```python
from build123d import *

# Parameters (mm, degrees)
CUT_SWEEP1_PITCH   = 0.793751588
CUT_EXTRUDE1_DEPTH = 1.955803912
FILLET1_R          = 0.30480061
FILLET2_R          = 0.396875794
CHAMFER3_SIZE      = 0.127


with BuildPart() as part:
    # Sketch1 → Revolve1 (revolve)
    with BuildSketch(Plane.XY, mode=Mode.PRIVATE) as revolve1_sk:
        Polygon((0, 0), (0, 29.565608331), (2.082804166, 29.565608331), (2.082804166, 4.165608331), (3.429006858, 4.165608331), (3.429006858, 0), align=None)
    revolve(revolve1_sk.sketch.rotate(Axis((0, 0, 0), (0, 1, 0)), 90), axis=Axis((0, 0, 0), (0, 1, 0)))

    # Cut-Sweep1: arcs per turn and ends read off the stored shape
    # Cut-Sweep1: the profile of Sketch3 profile screwed along a right-hand helix through 4.999992 turns, 8 arcs to a turn; built about Z, then put on its axis
    cut_sweep1_z = Axis((0, 0, 0), (0, 0, 1))
    cut_sweep1_corners = [(2.083104166, 0, -0.595163691), (2.083104166, 0, -0.992339484), (1.685928372, 0, -0.793751588)]
    with BuildLine(mode=Mode.PRIVATE) as cut_sweep1_profile:
        Line(cut_sweep1_corners[0], cut_sweep1_corners[1])
        Line(cut_sweep1_corners[1], cut_sweep1_corners[2])
        Line(cut_sweep1_corners[2], cut_sweep1_corners[0])
    cut_sweep1_cap = Face(cut_sweep1_profile.wire())
    cut_sweep1_turn_angles = [0, 22.5, 45, 67.5, 90, 112.5, 135, 157.5, 180, 202.5, 225, 247.5, 270, 292.5, 315, 337.5, 360]
    cut_sweep1_turn_weights = [1, 0.9238795325112867, 1, 0.9238795325112867, 1, 0.9238795325112867, 1, 0.9238795325112867, 1, 0.9238795325112867, 1, 0.9238795325112867, 1, 0.9238795325112867, 1, 0.9238795325112867, 1]
    cut_sweep1_turn_rails = [Edge.make_bspline([Vector(p[0], p[1], 0).rotate(cut_sweep1_z, cut_sweep1_turn_angles[k]) / cut_sweep1_turn_weights[k] + Vector(0, 0, p[2] + CUT_SWEEP1_PITCH * cut_sweep1_turn_angles[k] / 360) for k in range(17)], [0, 0, 0, 1, 1, 2, 2, 3, 3, 4, 4, 5, 5, 6, 6, 7, 7, 8, 8, 8], 2, cut_sweep1_turn_weights) for p in cut_sweep1_corners]
    cut_sweep1_turn_sides = [Face.make_surface_from_curves(cut_sweep1_turn_rails[p[0]], cut_sweep1_turn_rails[p[1]]) for p in [(0, 1), (1, 2), (2, 0)]]
    cut_sweep1_last_angles = [1440, 1462.5, 1485, 1507.5, 1530, 1552.5, 1575, 1597.5, 1620, 1642.5, 1665, 1687.5, 1710, 1732.5, 1755, 1777.4985, 1799.997]
    cut_sweep1_last_weights = [1, 0.9238795325112867, 1, 0.9238795325112867, 1, 0.9238795325112867, 1, 0.9238795325112867, 1, 0.9238795325112867, 1, 0.9238795325112867, 1, 0.9238795325112867, 1, 0.9238895508235082, 1]
    cut_sweep1_last_rails = [Edge.make_bspline([Vector(p[0], p[1], 0).rotate(cut_sweep1_z, cut_sweep1_last_angles[k]) / cut_sweep1_last_weights[k] + Vector(0, 0, p[2] + CUT_SWEEP1_PITCH * cut_sweep1_last_angles[k] / 360) for k in range(17)], [0, 0, 0, 1, 1, 2, 2, 3, 3, 4, 4, 5, 5, 6, 6, 7, 7, 8, 8, 8], 2, cut_sweep1_last_weights) for p in cut_sweep1_corners]
    cut_sweep1_last_sides = [Face.make_surface_from_curves(cut_sweep1_last_rails[p[0]], cut_sweep1_last_rails[p[1]]) for p in [(0, 1), (1, 2), (2, 0)]]
    cut_sweep1 = Plane(origin=(0, 29.565608331, 0), x_dir=(0, 0, 1), z_dir=(0, -1, 0)) * Solid(Shell([*[p.moved(Location((0, 0, CUT_SWEEP1_PITCH * i))) for i in range(4) for p in cut_sweep1_turn_sides], *cut_sweep1_last_sides, cut_sweep1_cap, cut_sweep1_cap.rotate(cut_sweep1_z, 1799.997).moved(Location((0, 0, CUT_SWEEP1_PITCH * 1799.997 / 360)))]))
    add(cut_sweep1, mode=Mode.SUBTRACT)

    # Sketch4 → Cut-Extrude1 (cut)
    with BuildSketch(Plane(origin=(0, 0, 0), x_dir=(1, 0, 0), z_dir=(0, 1, 0))):
        Polygon((0, 2.06772639), (-1.790703581, 1.033863195), (-1.790703581, -1.033863195), (0, -2.06772639), (1.790703581, -1.033863195), (1.790703581, 1.033863195), align=None)
    extrude(amount=CUT_EXTRUDE1_DEPTH, mode=Mode.SUBTRACT)

    # Fillet1
    fillet1_edges = [part.edges().sort_by_distance(p)[0] for p in [
        (0, 4.165608331, 2.082804166),
    ]]
    fillet(fillet1_edges, radius=FILLET1_R)

    # Fillet2
    fillet2_edges = [part.edges().sort_by_distance(p)[0] for p in [
        (1.790703581, 0.977901956, -1.033863195),
        (0, 0.977901956, -2.06772639),
        (-1.790703581, 0.977901956, -1.033863195),
        (-1.790703581, 0.977901956, 1.033863195),
        (0, 0.977901956, 2.06772639),
        (1.790703581, 0.977901956, 1.033863195),
        (0.895351791, 1.955803912, -1.550794792),
        (-0.895351791, 1.955803912, -1.550794792),
        (-1.790703581, 1.955803912, 0),
        (-0.895351791, 1.955803912, 1.550794792),
        (0.895351791, 1.955803912, 1.550794792),
        (1.790703581, 1.955803912, 0),
    ]]
    fillet(fillet2_edges, radius=FILLET2_R)

    # Chamfer1: read off the stored shape, not the designer's step
    # Chamfer1 outline → Chamfer1 (revolve, cut)
    with BuildSketch(Plane.XY):
        Polygon((2.082804166, 29.565608331), (1.879603759, 29.565608331), (2.082804166, 29.236469354), align=None)
    revolve(axis=Axis((0, 0, 0), (0, 1, 0)), mode=Mode.SUBTRACT)

    # Chamfer2: read off the stored shape, not the designer's step
    # Chamfer2 outline → Chamfer2 (revolve, cut)
    with BuildSketch(Plane.XY):
        Polygon((2.853013648, 0), (3.429006858, 0), (3.429006858, 0.355600711), align=None)
        Polygon((3.073406147, 4.165608331), (3.429006858, 3.589615121), (3.429006858, 4.165608331), align=None)
    revolve(axis=Axis((0, 0, 0), (0, 1, 0)), mode=Mode.SUBTRACT)

    # Chamfer3
    chamfer3_edges = [part.edges().sort_by_distance(p)[0] for p in [
        (0.895351791, 0, -1.550794792),
        (-0.895351791, 0, -1.550794792),
        (-1.790703581, 0, 0),
        (-0.895351791, 0, 1.550794792),
        (0.895351791, 0, 1.550794792),
        (1.790703581, 0, 0),
        (0, 0, -2.006329491),
        (1.737532307, 0, -1.003164745),
        (1.737532307, 0, 1.003164745),
        (0, 0, 2.006329491),
        (-1.737532307, 0, 1.003164745),
        (-1.737532307, 0, -1.003164745),
    ]]
    chamfer(chamfer3_edges, length=CHAMFER3_SIZE)


solid = part.part
```
For this review, take the finished solid that the model builds, in its own axes (mm). A direction names the side the tool comes from. Coordinates: 2 decimals unless noted, no trailing zeros. Loops run counter-clockwise (first coordinate to the right, second up) from the corner with the lowest first, then second, coordinate; pieces in that order, holes last. Notation, with made-up numbers: (57.5, 47) -> (94.5, 47) arc R21 ccw to (94.5, 55) -> close; hole circle Ø10 at (81, -39). An arc over 180 degrees is marked (long way). Return JSON: item names as keys, results as strings. Group by question number.
(1) Consider section A-A, the plane y = 19. Give the boundary of the cut face in (x, z), plus the area to 3 significant figures.
(2) Mouldability with a two-part tool opening along X and no side actions: class faces 1 (the flat face through (-0.905, 0.833, 1.545)), 2 (the flat face through (-1, 0, -2)) as pulls with the +X half, pulls with the -X half, needs draft (parallel to the pull), parting line crosses it, or undercut.
(3) For pin 1 Ø2 at (x, y) = (-2.5, 20) entering from +Z (3 decimals); pin 2 Ø3 at (x, y) = (-2, 13) entering from -Z; pin 3 Ø0.8 at (x, z) = (-0.5, -0.5) entering from -Y, all flat-tipped, find the tip position at first contact; note any pin that passes through.
(4) Tool access review of faces 3 (the flat face through (0, 29.566, 0)), 4 (the cylindrical face through (-0.829, 1.836, 1.458)), 5 (the flat face through (2, 4.166, 2)): name each direction out of +Z, -Z, +X, -X, +Y, -Y from which nothing blocks a thin tool from reaching the whole face with its end or side.
(5) To check wall thickness, follow L1, parallel to Y at x = 2.5, z = 0; L2, parallel to Z at x = 3, y = 2.5; L3, parallel to X at y = 27.5, z = 0.5. State the ranges of each line that lie inside material, in increasing order.
Results below:
{
 "1": {"outline": "circle Ø4.17 at (0, 0)", "area": "13.6 mm2"},
 "2": {"face 1": "undercut", "face 2": "needs draft"},
 "3": {"pin 1": "stops at z = 1.445", "pin 2": "stops at z = -2.02", "pin 3": "stops at y = 1.96"},
 "4": {"face 3": "+Z, -Z, +X, -X, +Y", "face 4": "-Y", "face 5": "+Y"},
 "5": {"L1": "y = 0 to 4.17", "L2": "z = -1.66 to 1.66", "L3": "x = -2.02 to 1.92"}
}
